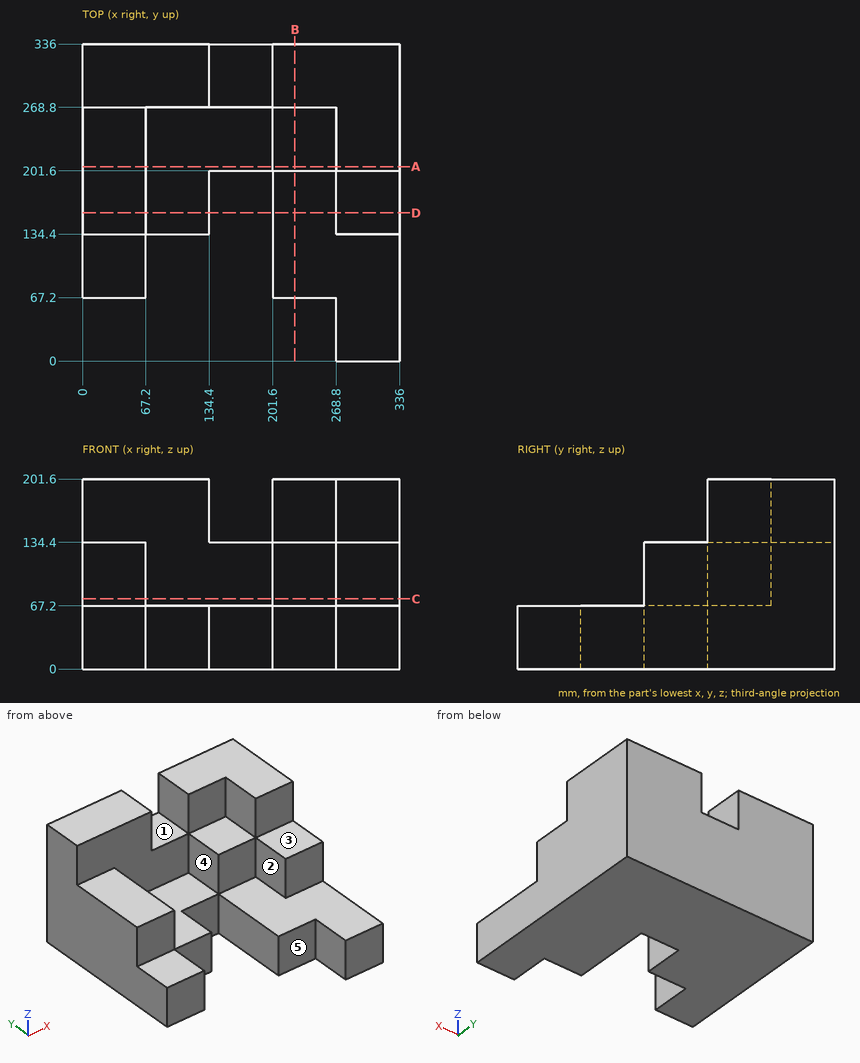
Geometry: see drawing. Coordinates: mm, zero at the bounding-box minimum. A direction names the side the tool comes from. Round coordinates to 2 decimals unless told otherwise and drop trailing zeros. Write each loop counter-clockwise with the first axis right and the second up, starting at its lowest first coordinate (ties: lowest second). Pieces come first, ordered by that corner, then holes. Notation, with made-up numbers: (45, 78) - (86, 78) arc R20 cw to (86, 84) - close; hole circle Ø9 at (32.5, 89). An arc over 180 degrees is marked (long way). Use CSV: the item, a comma, the result in double quotes. Start each with the question number.
(1) First-contact query: pin 1 Ø10 at (x, z) = (111.5, 113) entering from -Y; pin 2 Ø5 at (x, y) = (128, 241.5) entering from +Z; pin 3 Ø20 at (x, y) = (233, 239.5) entering from +Z. Flat tips, straight axial feed; report the tip coordinate or a pass-through.
(2) Material intervals for probe 1 along X at (y, z) = (182, 46.5); probe 2 along Y at (x, z) = (53, 94.5); probe 3 along Y at (x, z) = (229, 178), sorted ascending. Write a range as [from, to].
(3) Set-up query: the marked faces 1, 2 and 3. Return all of +Z, -Z, +X, -X, +Y, -Y with unobstructed straight access to the full face (end or side cutting, diameter ignored); none if empty.
(4) Cut plane B-B, the plane x = 225. Return loops of the section in (y, z).
(5) Cut plane C-C, the plane z = 74.5. Return loops of the section in (x, y), and give its area (3 significant figures).
(6) Cut plane A-A, the plane y = 206. Return loops of the section in (x, z), and give its area (3 significant figures).
(7) Mould query, pull axis X, two halves, no side actions, for the marked faces 4 and 5. Classes: pulls with the +X half, pulls with the -X half, needs draft (parallel to the pull), parting line crosses it, or undercut.
(8) Cut plane D-D, the plane y = 157. Return loops of the section in (x, z), and give its area (3 significant figures).
Geometry says:
1,pin 1,"y = 268.8"
1,pin 2,"z = 67.2"
1,pin 3,"z = 134.4"
2,probe 1,"[0, 134.4], [201.6, 336]"
2,probe 2,"[134.4, 336]"
2,probe 3,"[268.8, 336]"
3,face 1,"+Z, +Y, -Y"
3,face 2,"+Z, -Y"
3,face 3,"+Z, +X, -X, -Y"
4,outline,"(67.2, 0) - (336, 0) - (336, 201.6) - (268.8, 201.6) - (268.8, 134.4) - (201.6, 134.4) - (201.6, 67.2) - (67.2, 67.2) - close"
5,outline,"(0, 134.4) - (67.2, 134.4) - (67.2, 268.8) - (201.6, 268.8) - (201.6, 201.6) - (268.8, 201.6) - (268.8, 134.4) - (336, 134.4) - (336, 336) - (0, 336) - close"
5,area,"45,200 mm²"
6,outline,"(0, 0) - (336, 0) - (336, 201.6) - (268.8, 201.6) - (268.8, 134.4) - (201.6, 134.4) - (201.6, 67.2) - (67.2, 67.2) - (67.2, 134.4) - (0, 134.4) - close"
6,area,"40,600 mm²"
7,face 4,"undercut"
7,face 5,"needs draft"
8,outline,"(0, 0) - (134.4, 0) - (134.4, 67.2) - (67.2, 67.2) - (67.2, 134.4) - (0, 134.4) - close; (201.6, 0) - (336, 0) - (336, 134.4) - (268.8, 134.4) - (268.8, 67.2) - (201.6, 67.2) - close"
8,area,"27,100 mm²"
